from build123d import *

# Parameters (mm, degrees)
BOSS_EXTRUDE1_DEPTH     = 28
CUT_EXTRUDE1_DEPTH      = 124.299913301
CUT_EXTRUDE1_DEPTH_BACK = 124.299913301
SKETCH2_R               = 15


with BuildPart() as part:
    # Sketch1 → Boss-Extrude1 (new body)
    with BuildSketch(Plane(origin=(0, 0, 0), x_dir=(1, 0, 0), z_dir=(0, 1, 0))):
        with BuildLine():
            Line((34.09833793, -47.060053749), (48.497353619, -71.9998805))
            ThreePointArc((48.497353619, -71.9998805), (54.23905714, -67.779796256), (59.615306076, -63.103021968))
            ThreePointArc((59.615306076, -63.103021968), (60.621778265, -35), (84.456473118, -20.076858532))
            ThreePointArc((84.456473118, -20.076858532), (85.818553991, -13.082503233), (86.602402392, -6))
            Line((86.602402392, -6), (57.804371015, -6))
            ThreePointArc((57.804371015, -6), (51.804371015, 0), (57.804371015, 6))
            Line((57.804371015, 6), (86.602402392, 6))
            ThreePointArc((86.602402392, 6), (85.818553991, 13.082503233), (84.456473118, 20.076858532))
            ThreePointArc((84.456473118, 20.076858532), (60.621778265, 35), (59.615306076, 63.103021968))
            ThreePointArc((59.615306076, 63.103021968), (54.23905714, 67.779796256), (48.497353619, 71.9998805))
            Line((48.497353619, 71.9998805), (34.09833793, 47.060053749))
            ThreePointArc((34.09833793, 47.060053749), (25.902185507, 44.863901326), (23.706033085, 53.060053749))
            Line((23.706033085, 53.060053749), (38.105048773, 77.9998805))
            ThreePointArc((38.105048773, 77.9998805), (31.579496851, 80.862299489), (24.841167042, 83.1798805))
            ThreePointArc((24.841167042, 83.1798805), (0, 70), (-24.841167042, 83.1798805))
            ThreePointArc((-24.841167042, 83.1798805), (-31.579496851, 80.862299489), (-38.105048773, 77.9998805))
            Line((-38.105048773, 77.9998805), (-23.706033085, 53.060053749))
            ThreePointArc((-23.706033085, 53.060053749), (-25.902185507, 44.863901326), (-34.09833793, 47.060053749))
            Line((-34.09833793, 47.060053749), (-48.497353619, 71.9998805))
            ThreePointArc((-48.497353619, 71.9998805), (-54.23905714, 67.779796256), (-59.615306076, 63.103021968))
            ThreePointArc((-59.615306076, 63.103021968), (-60.621778265, 35), (-84.456473118, 20.076858532))
            ThreePointArc((-84.456473118, 20.076858532), (-85.818553991, 13.082503233), (-86.602402392, 6))
            Line((-86.602402392, 6), (-57.804371015, 6))
            ThreePointArc((-57.804371015, 6), (-51.804371015, 0), (-57.804371015, -6))
            Line((-57.804371015, -6), (-86.602402392, -6))
            ThreePointArc((-86.602402392, -6), (-85.818553991, -13.082503233), (-84.456473118, -20.076858532))
            ThreePointArc((-84.456473118, -20.076858532), (-60.621778265, -35), (-59.615306076, -63.103021968))
            ThreePointArc((-59.615306076, -63.103021968), (-54.23905714, -67.779796256), (-48.497353619, -71.9998805))
            Line((-48.497353619, -71.9998805), (-34.09833793, -47.060053749))
            ThreePointArc((-34.09833793, -47.060053749), (-25.902185507, -44.863901326), (-23.706033085, -53.060053749))
            Line((-23.706033085, -53.060053749), (-38.105048773, -77.9998805))
            ThreePointArc((-38.105048773, -77.9998805), (-31.579496851, -80.862299489), (-24.841167042, -83.1798805))
            ThreePointArc((-24.841167042, -83.1798805), (0, -70), (24.841167042, -83.1798805))
            ThreePointArc((24.841167042, -83.1798805), (31.579496851, -80.862299489), (38.105048773, -77.9998805))
            Line((38.105048773, -77.9998805), (23.706033085, -53.060053749))
            ThreePointArc((23.706033085, -53.060053749), (25.902185507, -44.863901326), (34.09833793, -47.060053749))
        make_face()
    extrude(amount=BOSS_EXTRUDE1_DEPTH)

    # Sketch2 → Cut-Extrude1 (cut, two sides: drawn at the far end of the back side and taken through both)
    with BuildSketch(Plane(origin=(0, 28, 0), x_dir=(1, 0, 0), z_dir=(0, 1, 0)).offset(-CUT_EXTRUDE1_DEPTH_BACK)):
        with Locations(Location((0, 0, 0), (0, 0, 270))):
            Circle(SKETCH2_R)
    extrude(amount=CUT_EXTRUDE1_DEPTH + CUT_EXTRUDE1_DEPTH_BACK, mode=Mode.SUBTRACT)


solid = part.part
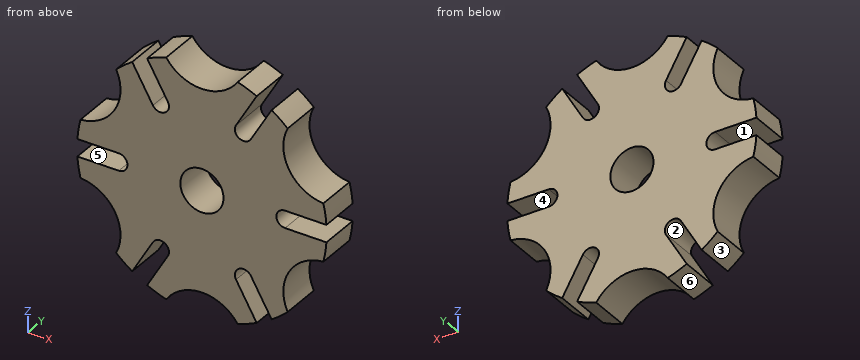
CAD build for the part. Positions are in the model's coordinates, mm. Face numbers are marked on the shaded views. A direction names the side the tool comes from. Round coordinates to 2 decimals unless told otherwise and drop trailing zeros. Loops run counter-clockwise (first coordinate to the right, second up) from the corner with the lowest first, then second, coordinate; pieces in that order, holes last.
(1) Wall check: line 1 along X through (y, z) = (16.25, 0); line 2 along Z through (x, y) = (-13, 2); line 3 along Z through (x, y) = (7, 18.25). Give the ranges that are in metal, low to high.
(2) Drop flat-ended pins along their axis: pin 1 (8.5 mm diameter, centred on x = 68.5, y = 10, fed in from +Z); pin 2 (3 mm diameter, centred on x = 5, z = -22.5, fed in from -Y); pin 3 (14 mm diameter, centred on x = -68.5, y = 15, fed in from -Z); pin 4 (8 mm diameter, centred on x = 31.5, y = 3.5, fed in from -Z). Give the stop position or say it passes through.
(3) Cut at A-A (z = 0). Give the cut face in (x, y).
(4) Cut at D-D (x = -46). Give the cut face in (y, z).
(5) Cut at C-C (z = -51). Give the cut face in (x, y), plus the area to 3 significant figures.
(6) Two-plate mould, pull along X, no slides. Class the marked faces 1, 2 and 3: +X half, -X half, draft (parallel to the pull), parting line (faces both ways), or undercut.
(7) Cut at B-B (x = 0). Give the cut face in (y, z), plus the area to 3 significant figures.
(8) Which spindle directions (+Z, -Z, +X, -X, +Y, -Y) get a long thin tool onto all of the face, cutting with end or side? Do the marked faces 4, 5 and 6. Say none if no direction does.
Findings below:
1. line 1: x = -51.8 to -15, 15 to 51.8
1. line 2: z = -72.96 to -7.48, 7.48 to 72.96
1. line 3: z = -70.83 to -13.27, 13.27 to 70.83
2. pin 1: stops at z = 29.99
2. pin 2: stops at y = 0
2. pin 3: stops at z = -33.57
2. pin 4: stops at z = -82.34
3. outline: (-51.8, 0) - (-15, 0) - (-15, 28) - (-51.8, 28) - close; (15, 0) - (51.8, 0) - (51.8, 28) - (15, 28) - close
4. outline: (0, -67.67) - (28, -67.67) - (28, 67.67) - (0, 67.67) - close
5. outline: (-56.62, 0) - (-36.37, 0) - (-36.37, 28) - (-56.62, 28) - close; (-22.98, 0) - (22.98, 0) - (22.98, 28) - (-22.98, 28) - close; (36.37, 0) - (56.62, 0) - (56.62, 28) - (36.37, 28) - close
5. area: 2,420 mm2
6. face 1: draft
6. face 2: undercut
6. face 3: -X half
7. outline: (0, -70) - (28, -70) - (28, -15) - (0, -15) - close; (0, 15) - (28, 15) - (28, 70) - (0, 70) - close
7. area: 3,080 mm2
8. face 4: +X, +Y, -Y
8. face 5: -X, +Y, -Y
8. face 6: -Z, -X, +Y, -Y
